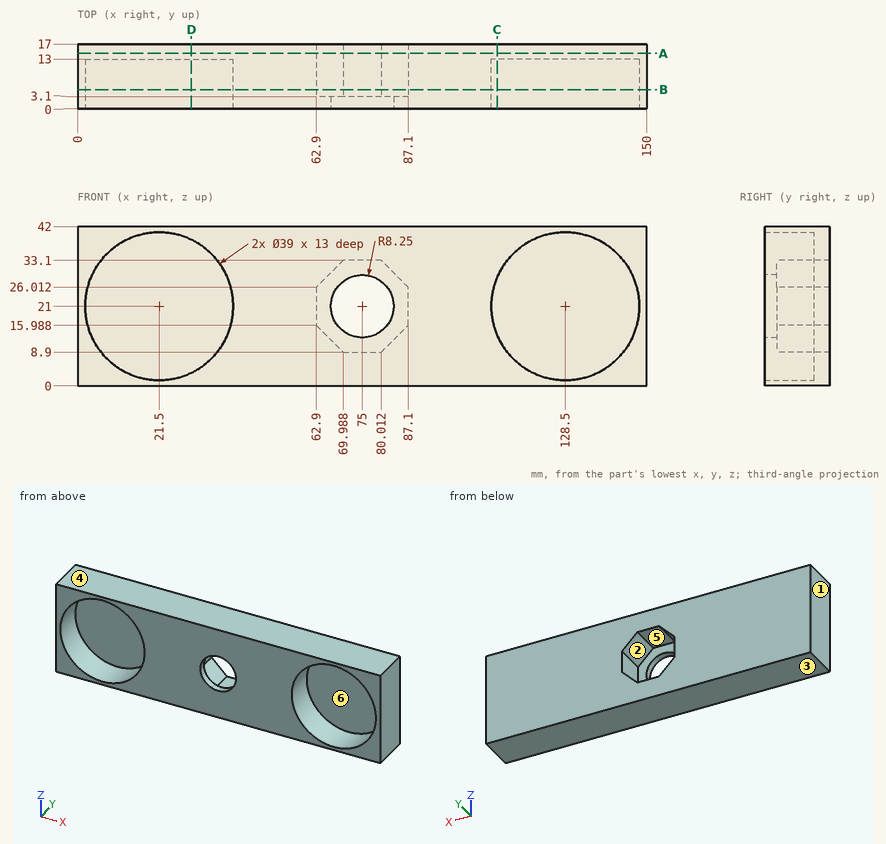
Geometry: see drawing. Coordinates: mm, zero at the bounding-box minimum. A direction names the side the tool comes from. Round coordinates to 2 decimals unless told otherwise and drop trailing zeros. Loops run counter-clockwise (first coordinate to the right, second up) from the corner with the lowest first, then second, coordinate; pieces in that order, holes last. Notation, with made-up numbers: (-5.75, 74) - (18.25, 74) arc R25 ccw to (18.25, 104) - close; hole circle Ø4 at (22, 8). An arc over 180 degrees is marked (long way). One line per item, written item: value. Start each with the question number.
(1) Draft query along X for the marked faces 1, 2 and 3. Return one class per face: +X half, -X half, draft (parallel to the pull), parting line (faces both ways), or undercut.
(2) Access query for the marked faces 4, 5 and 6. Directions: +Z, -Z, +X, -X, +Y, -Y. A direction counts if a zero-diameter tool reaches every point of the face in a straight line with its end or side. Return the directions, or none.
(3) Section B-B, the plane y = 5. Return loops of the section in (x, z), plus the area to 3 significant figures.
(4) Contact query for flat-ended pins moving along their axis: P1, Ø7.5, axis at x = 80, z = 17, coming from the +Y side; P2, Ø23.5, axis at x = 128.5, z = 21, coming from the -Y side. Output: stop coordinate, or through.
(5) Section A-A, the plane y = 14.5. Return loops of the section in (x, z).
(6) Section D-D, the plane x = 30. Return loops of the section in (y, z).
(7) Ray query, line 1 (X direction, y = 7, z = 21); line 2 (Z direction, x = 21.5, y = 5); line 3 (X direction, y = 11.5, z = 19). Return the intervals inside material, ascending. Write a range as [from, to].
(8) Section C-C, the plane x = 110.5. Return loops of the section in (y, z), plus the area to 3 significant figures.
Results below:
1. face 1: -X half
1. face 2: undercut
1. face 3: draft
2. face 4: +Z, +X, -X, +Y, -Y
2. face 5: +Y
2. face 6: -Y
3. outline: (0, 0) - (150, 0) - (150, 42) - (0, 42) - close; hole circle Ø39 at (21.5, 21); hole (62.9, 15.99) - (69.99, 8.9) - (80.01, 8.9) - (87.1, 15.99) - (87.1, 26.01) - (80.01, 33.1) - (69.99, 33.1) - (62.9, 26.01) - close; hole circle Ø39 at (128.5, 21)
3. area: 3,430 mm^2
4. P1: y = 3.1
4. P2: y = 13
5. outline: (0, 0) - (150, 0) - (150, 42) - (0, 42) - close; hole (62.9, 15.99) - (69.99, 8.9) - (80.01, 8.9) - (87.1, 15.99) - (87.1, 26.01) - (80.01, 33.1) - (69.99, 33.1) - (62.9, 26.01) - close
6. outline: (0, 0) - (17, 0) - (17, 42) - (0, 42) - (0, 38.55) - (13, 38.55) - (13, 3.45) - (0, 3.45) - close
7. line 1: [0, 2], [41, 62.9], [87.1, 109], [148, 150]
7. line 2: [0, 1.5], [40.5, 42]
7. line 3: [0, 2.1], [40.9, 62.9], [87.1, 109.1], [147.9, 150]
8. outline: (0, 0) - (17, 0) - (17, 42) - (0, 42) - (0, 28.5) - (13, 28.5) - (13, 13.5) - (0, 13.5) - close
8. area: 519 mm^2
